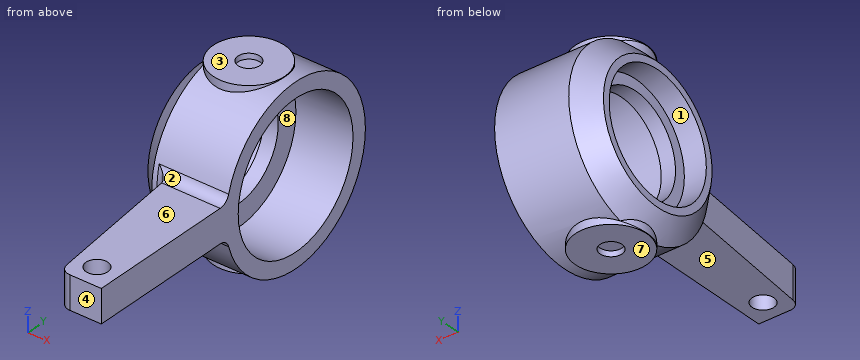
from build123d import *

# Parameters (mm, degrees)
F0_R         = 7.9
F1_DEPTH     = 4.25
F2_R         = 3.25
F3_DEPTH     = 7.95
F4_R         = 6.5
F5_DEPTH     = 5.2
F6_R         = 5.5
F7_DEPTH     = 2
F8_R         = 4.5
F9_DEPTH     = 8.5010001
F10_S5_R     = 3.25
F10_T6_DEPTH = 13
F12_DEPTH    = 1.5
F13_R        = 1
F14_R        = 1
F15_DEPTH    = 0.5
F16_R        = 1
F17_DEPTH    = 4
F18_R        = 1


# Not quite as in the source:
# - a fillet or chamfer that OpenCascade refuses, or shapes differently, is made with other operations: its cross-section is extruded or revolved along the edge and cut away or added
# - a pattern or mirror of a feature is missing from the dataset's text; its kind, count and spacing are read off the source's solid


with BuildPart() as f1:
    # F0 (on Right) → F1 (new body, symmetric)
    with BuildSketch(Plane.YZ):
        Circle(F0_R)
    extrude(amount=F1_DEPTH, both=True)

    # F2 (on Top) → F3 (join, symmetric)
    with BuildSketch(Plane.XY):
        Circle(F2_R)
    extrude(amount=F3_DEPTH, both=True)

    # F4 (on face) → F5 (cut)
    with BuildSketch(Plane.YZ.offset(4.25)):
        Circle(F4_R)
    extrude(amount=-F5_DEPTH, mode=Mode.SUBTRACT)

    # F6 (on face) → F7 (cut)
    with BuildSketch(Plane(origin=(-4.25, 0, 0), x_dir=(0, -1, 0), z_dir=(-1, 0, 0))):
        Circle(F6_R)
    extrude(amount=-F7_DEPTH, mode=Mode.SUBTRACT)

    # F8 (on face) → F9 (cut, through all)
    with BuildSketch(Plane.YZ.offset(4.25)):
        Circle(F8_R)
    extrude(amount=-F9_DEPTH, mode=Mode.SUBTRACT)

    # F10: chamfer of 1.75 on 1 edges, made by hand


with BuildPart() as f10_tool2:
    # F10_s3 → F10_t4 (revolve)
    with BuildSketch(Plane.XY):
        Polygon((-2.5, 7.9), (-4.25, 6.15), (-4.25, 7.9), align=None)
    revolve(axis=Axis((-4.25, 0, 0), (1, 0, 0)))

    # F10_s5 → F10_t6 (cut, symmetric)
    with BuildSketch(Plane.XY):
        Circle(F10_S5_R)
    extrude(amount=F10_T6_DEPTH, both=True, mode=Mode.SUBTRACT)


with BuildPart() as f1_1:
    add(f1.part)

    # F10_t1: cut F10_tool2
    add(f10_tool2.part, mode=Mode.SUBTRACT)

    # F11 (on Top) → F12 (join, symmetric)
    with BuildSketch(Plane.XY):
        Polygon((-1.25, -7), (0.5, -22), (4.25, -22), (4.25, -7), align=None)
    extrude(amount=F12_DEPTH, both=True)

    # F13
    f13_edges = [f1_1.edges().sort_by_distance(p)[0] for p in [
        (-1.145, -7.9, 0),
        (1.544117, -7.756288, 1.5),
        (1.544117, -7.756288, -1.5),
    ]]
    fillet(f13_edges, radius=F13_R)

    # F14 (on face) → F15 (cut)
    with BuildSketch(Plane.XY.offset(7.95)):
        Circle(F14_R)
    f15 = extrude(amount=-F15_DEPTH, mode=Mode.SUBTRACT)

    # F15_copies: F15 across plane
    add(f15.mirror(Plane(origin=(0, 0, 0), x_dir=(-1, 0, 0), z_dir=(0, 0, -1))), mode=Mode.SUBTRACT)

    # F16 (on Top) → F17 (cut, symmetric)
    with BuildSketch(Plane.XY):
        with Locations((2.25, -20)):
            Circle(F16_R)
    extrude(amount=F17_DEPTH, both=True, mode=Mode.SUBTRACT)

    # F18
    f18_edges = [f1_1.edges().sort_by_distance(p)[0] for p in [
        (0.5, -22, 0),
    ]]
    fillet(f18_edges, radius=F18_R)


solid = f1_1.part
Build history of the part. All positions in model axes, mm. Face numbers are marked on the shaded views. A direction names the side the tool comes from. Round coordinates to 2 decimals unless told otherwise and drop trailing zeros. Write each loop counter-clockwise with the first axis right and the second up, starting at its lowest first coordinate (ties: lowest second). Pieces come first, ordered by that corner, then holes. Notation, with made-up numbers: M 46.5,-28 L 89.5,-28 A17 ccw 89.5,-8 Z; hole C 57.25,78.25 d3. An arc over 180 degrees is marked long. Answer in a Markdown table with one row per item.
1. Probe L1, parallel to Y at x = 0, z = -7.7; L2, parallel to Z at x = 3, y = 0; L3, parallel to Y at x = 2.25, z = -0.65. List the from-to ranges inside material, lowest first. Write a range as [from, to].
Geometry check:
| item | result |
|---|---|
| L1 | [-3.25, -1], [1, 3.25] |
| L2 | [-7.95, -6.5], [6.5, 7.95] |
| L3 | [-22, -21], [-19, -6.47], [6.47, 7.87] |
2. Saw through at D-D (z = 0). State how many separate pieces and enclosed holes the cut face has, and give its area (3 significant figures).
Geometry check:
| item | result |
|---|---|
| separate pieces | 2 |
| enclosed holes | 1 |
| area | 91.3 mm2 |
3. Saw through at B-B (y = -20). List the corners of the cut face in (x, z).
Geometry check:
| item | result |
|---|---|
| outline | M 0.27,-1.5 L 1.25,-1.5 L 1.25,1.5 L 0.27,1.5 Z; M 3.25,-1.5 L 4.25,-1.5 L 4.25,1.5 L 3.25,1.5 Z |
4. Flat gauge pins, fed straight in: P1, Ø0.6, axis at x = 0, y = 0, coming from the -Z side; P2, Ø3, axis at x = 2.25, y = -20, coming from the +Z side; P3, Ø0.6, axis at x = 0, y = 0, coming from the +Z side. Where does each tip first touch, or does it go through?
Geometry check:
| item | result |
|---|---|
| P1 | z = -7.45 |
| P2 | z = 1.5 |
| P3 | z = 7.45 |
5. Saw through at A-A (x = 2.25). List the corners of the cut face in (y, z).
Geometry check:
| item | result |
|---|---|
| outline | M -22,-1.5 L -21,-1.5 L -21,1.5 L -22,1.5 Z; M -19,-1.5 L -8.54,-1.5 A1 cw -7.58,-2.22 A7.9 ccw -2.35,-7.54 L -2.35,-7.95 L 2.35,-7.95 L 2.35,-7.54 A7.9 ccw 2.35,7.54 L 2.35,7.95 L -2.35,7.95 L -2.35,7.54 A7.9 ccw -7.58,2.22 A1 cw -8.54,1.5 L -19,1.5 Z; hole C 0,0 d13 |
6. Saw through at C-C (x = 0). List the corners of the cut face in (y, z), and give its area (3 significant figures).
Geometry check:
| item | result |
|---|---|
| outline | M -17.71,-1.5 L -8.54,-1.5 A1 cw -7.58,-2.22 A7.9 ccw -3.25,-7.2 L -3.25,-7.95 L -1,-7.95 L -1,-7.45 L 1,-7.45 L 1,-7.95 L 3.25,-7.95 L 3.25,-7.2 A7.9 ccw 3.25,7.2 L 3.25,7.95 L 1,7.95 L 1,7.45 L -1,7.45 L -1,7.95 L -3.25,7.95 L -3.25,7.2 A7.9 ccw -7.58,2.22 A1 cw -8.54,1.5 L -17.71,1.5 Z; hole C 0,0 d13 |
| area | 94.8 mm2 |
7. Mould opens along Y. For the marked faces 1, 2 and 3 say: +Y half, -Y half, draft (parallel to the pull), parting line (faces both ways), or undercut.
Geometry check:
| item | result |
|---|---|
| face 1 | undercut |
| face 2 | -Y half |
| face 3 | draft |
8. Which spindle directions (+Z, -Z, +X, -X, +Y, -Y) get a long thin tool onto all of the face, cutting with end or side? Do the marked faces 4, 5, 6, 7 and 8. Say none if no direction does.
Geometry check:
| item | result |
|---|---|
| face 4 | +Z, -Z, +X, -X, -Y |
| face 5 | -Z, +X, -X, -Y |
| face 6 | +Z, +X, -X, -Y |
| face 7 | -Z, +X, -X, +Y, -Y |
| face 8 | +X |
